Input: part model. Units: mm. Frame: model coordinates. A direction names the side the tool comes from. Round coordinates to 2 decimals unless told otherwise and drop trailing zeros. Loops run counter-clockwise (first coordinate to the right, second up) from the corner with the lowest first, then second, coordinate; pieces in that order, holes last. Notation, with made-up numbers: (17.25, 31) -> (42.25, 31) arc R24 cw to (42.25, 52) -> close; hole circle Ø11 at (-13.75, -34.5). An arc over 180 degrees is marked (long way). Answer in a Markdown table with one row per item. Add a question column.
Q1. Section A-A, the plane z = 5.5. Output: boundary loops of the cut face in (x, y) (3 decimals).
Q2. Mould query, pull axis X, two halves, no side actions, for faces 4 (the face through (-12.74, -7.63, 4.08)), 5 (the face through (-4.336, -19.524, 7.395)), 6 (the face through (0, -18, 0)). Classes: pulls with the +X half, pulls with the -X half, needs draft (parallel to the pull), parting line crosses it, or undercut.
Q3. Reachability of faces 1 (the face through (0, 0, 10)), 2 (the face through (-5, 9, 15)), 3 (the face through (0, 0, 3)) from +Z, -Z, +X, -X, +Y, -Y: full face, straight path, thin tool, end or side. Return the list, or none.
Q4. Section B-B, the plane y = 0. Output: boundary loops of the cut face in (x, z).
Q5. Section C-C, the plane x = -8. Output: boundary loops of the cut face in (y, z).
Q6. Ray query, L1, parallel to X at y = -7.5, z = 7.5; L2, parallel to X at y = -8, z = 9.25; L3, parallel to Y at x = -13.5, z = 5.5. Return the intervals inside material, ascending. Write a range as from..to.
Q7. Section D-D, the plane z = 11.75. Output: boundary loops of the cut face in (x, y) (3 decimals), and give its area (3 significant figures).
Q8. Pin query (flat end, axial travel): pin 1 (4 mm diameter, centred on x = 0, y = -15, fed in from -Z); pin 2 (2 mm diameter, centred on x = 14, z = 11.5, fed in from -Y); pin 3 (4 mm diameter, centred on x = 14.5, z = 13, fed in from -Y). Return the tip coordinate at first contact, or that it passes through.
```python
from build123d import *

# Parameters (mm, degrees)
SKETCH1_R           = 20
BOSS_EXTRUDE1_DEPTH = 15
SKETCH2_R           = 10
CUT_EXTRUDE1_DEPTH  = 5
CIRPATTERN1_COUNT   = 6
SKETCH5_R           = 17.5
CUT_EXTRUDE3_DEPTH  = 3


with BuildPart() as part:
    # Sketch1 → Boss-Extrude1 (new body)
    with BuildSketch(Plane.XY):
        Circle(SKETCH1_R)
    extrude(amount=BOSS_EXTRUDE1_DEPTH)

    # Sketch2 → Cut-Extrude1 (cut)
    with BuildSketch(Plane.XY.offset(15)):
        Circle(SKETCH2_R)
    extrude(amount=-CUT_EXTRUDE1_DEPTH, mode=Mode.SUBTRACT)

    # Sketch4 → M4x0.7 Tapped Hole1 (revolve, cut)
    with BuildSketch(Plane(origin=(0, 15, 15), x_dir=(0, -1, 0), z_dir=(1, 0, 0))):
        Polygon((0, 0), (0, 11.091420021), (1.65, 10.1), (1.65, 0), align=None)
    m4x0_7_tapped_hole1 = revolve(axis=Axis((0, 15, 21.35), (0, 0, -1)), mode=Mode.SUBTRACT)

    # CirPattern1: M4x0.7 Tapped Hole1 ×6 about axis
    cirpattern1_axis = Axis((0, 0, 0), (0, 0, 1))
    for i in range(1, CIRPATTERN1_COUNT):
        add(m4x0_7_tapped_hole1.rotate(cirpattern1_axis, i * 360 / CIRPATTERN1_COUNT), mode=Mode.SUBTRACT)

    # Sketch5 → Cut-Extrude3 (cut)
    with BuildSketch(Plane(origin=(0, 0, 0), x_dir=(-1, 0, 0), z_dir=(0, 0, -1))):
        Circle(SKETCH5_R)
    extrude(amount=-CUT_EXTRUDE3_DEPTH, mode=Mode.SUBTRACT)


solid = part.part
```
Answer block:
| question | item | result |
|---|---|---|
| 1 | outline | circle Ø40 at (0, 0); hole circle Ø3.3 at (-12.99, -7.5); hole circle Ø3.3 at (-12.99, 7.5); hole circle Ø3.3 at (0, -15); hole circle Ø3.3 at (0, 15); hole circle Ø3.3 at (12.99, -7.5); hole circle Ø3.3 at (12.99, 7.5) |
| 2 | face 4 | undercut |
| 2 | face 5 | parting line crosses it |
| 2 | face 6 | needs draft |
| 3 | face 1 | +Z |
| 3 | face 2 | +Z, +X, -X, +Y, -Y |
| 3 | face 3 | -Z |
| 4 | outline | (-20, 0) -> (-17.5, 0) -> (-17.5, 3) -> (17.5, 3) -> (17.5, 0) -> (20, 0) -> (20, 15) -> (10, 15) -> (10, 10) -> (-10, 10) -> (-10, 15) -> (-20, 15) -> close |
| 5 | outline | (-18.33, 0) -> (-15.56, 0) -> (-15.56, 3) -> (15.56, 3) -> (15.56, 0) -> (18.33, 0) -> (18.33, 15) -> (6, 15) -> (6, 10) -> (-6, 10) -> (-6, 15) -> (-18.33, 15) -> close |
| 6 | L1 | -18.54..-14.64, -11.34..11.34, 14.64..18.54 |
| 6 | L2 | -18.33..-14.56, -11.42..11.42, 14.56..18.33 |
| 6 | L3 | -14.76..-9.07, -5.93..5.93, 9.07..14.76 |
| 7 | outline | circle Ø40 at (0, 0); hole circle Ø3.3 at (-12.99, -7.5); hole circle Ø3.3 at (-12.99, 7.5); hole circle Ø20 at (0, 0); hole circle Ø3.3 at (0, -15); hole circle Ø3.3 at (0, 15); hole circle Ø3.3 at (12.99, -7.5); hole circle Ø3.3 at (12.99, 7.5) |
| 7 | area | 891 mm^2 |
| 8 | pin 1 | z = 3 |
| 8 | pin 2 | y = -15.2 |
| 8 | pin 3 | y = -15.61 |
